Part model, mm, in its own coordinate system. Give positions to 0.01 mm unless a question says otherwise; leave off trailing zeros. Write each loop counter-clockwise with the first axis right and the second up, starting at its lowest first coordinate (ties: lowest second). Pieces come first, ordered by that corner, then holes. Notation, with made-up numbers: (33.5, -3.5) - (54.5, -3.5) arc R30 cw to (54.5, 20.5) - close; hole circle Ø10 at (-11, 26.5). An arc over 180 degrees is marked (long way). Answer as a JSON object with one key per item and string values. Group by question number.
```python
from build123d import *

# Parameters (mm, degrees)
CYLINDER009_R     = 3
CYLINDER009_DEPTH = 10
BOX003_W          = 32
BOX003_H          = 26
BOX003_DEPTH      = 5
CYLINDER008_R     = 16
CYLINDER008_DEPTH = 5


with BuildPart() as cilindro002:
    # Cylinder009 → Cylinder009 (new body)
    with BuildSketch(Plane(origin=(40, 37, 28), x_dir=(1, 0, 0), z_dir=(0, 0, 1))):
        Circle(CYLINDER009_R)
    extrude(amount=CYLINDER009_DEPTH)


with BuildPart() as cubo002:
    # Box003 → Box003 (new body)
    with BuildSketch(Plane(origin=(3, -8, 30), x_dir=(1, 0, 0), z_dir=(0, 0, 1))):
        with Locations((16, 13)):
            Rectangle(BOX003_W, BOX003_H)
    extrude(amount=BOX003_DEPTH)


with BuildPart() as tapa:
    # Cylinder008 → Cylinder008 (new body)
    with BuildSketch(Plane(origin=(19, 18, 30), x_dir=(1, 0, 0), z_dir=(0, 0, 1))):
        Circle(CYLINDER008_R)
    extrude(amount=CYLINDER008_DEPTH)

    # Fusion003: union Cubo002
    add(cubo002.part)


with BuildPart() as tapa_1:
    # Fusion003 placement: moved
    add(tapa.part.moved(Location((28, 40, 3))))

    # Cut010: cut Cilindro002
    add(cilindro002.part, mode=Mode.SUBTRACT)


solid = tapa_1.part
```
1) Band-saw the part on B-B (x = 39.5). List the corners of the cut face in (y, z), plus the area to 3 significant figures.
2) Band-saw the part on C-C (z = 36.95). List the corners of the cut face in (x, y), plus the area to 3 significant figures.
3) Probe line 1 (X direction, y = 37, z = 36.45); line 2 (Y direction, x = 40, z = 35.85); line 3 (Y direction, x = 41, z = 36.35). List the from-to ranges inside material, lowest first.
4) Mould opens along Y. For faces 1 (the cylindrical face through (47, 74, 35)), 2 (the flat face through (47, 53, 38)), 3 (the cylindrical face through (37.79, 39.03, 35.47)), 4 (the flat face through (47, 32, 35)) say: pulls with the +Y half, pulls with the -Y half, needs draft (parallel to the pull), parting line crosses it, or undercut.
5) Band-saw the part on A-A (y = 37). List the corners of the cut face in (x, z), plus the area to 3 significant figures.
6) Drop flat-ended pins along their axis: P1, Ø1.5, axis at x = 50, z = 35.5, coming from the +Y side; P2, Ø5.5, axis at x = 40, y = 37, coming from the +Z side. Give the stop position or say it passes through.
7) Band-saw the part on D-D (y = 65). List the corners of the cut face in (x, z).
Verdict:
{
 "1": {"outline": "(32, 33) - (34.04, 33) - (34.04, 38) - (32, 38) - close; (39.96, 33) - (72.13, 33) - (72.13, 38) - (39.96, 38) - close", "area": "171 mm2"},
 "2": {"outline": "(31, 32) - (63, 32) - (63, 58) arc R16 ccw to (31, 58) - close; hole circle Ø6 at (40, 37)", "area": "1,210 mm2"},
 "3": {"line 1": "31 to 37, 43 to 63", "line 2": "32 to 34, 40 to 72.39", "line 3": "32 to 34.17, 39.83 to 72.83"},
 "4": {"face 1": "pulls with the +Y half", "face 2": "needs draft", "face 3": "undercut", "face 4": "pulls with the -Y half"},
 "5": {"outline": "(31, 33) - (37, 33) - (37, 38) - (31, 38) - close; (43, 33) - (63, 33) - (63, 38) - (43, 38) - close", "area": "130 mm2"},
 "6": {"P1": "y = 73.84", "P2": "through"},
 "7": {"outline": "(32.61, 33) - (61.39, 33) - (61.39, 38) - (32.61, 38) - close"}
}
